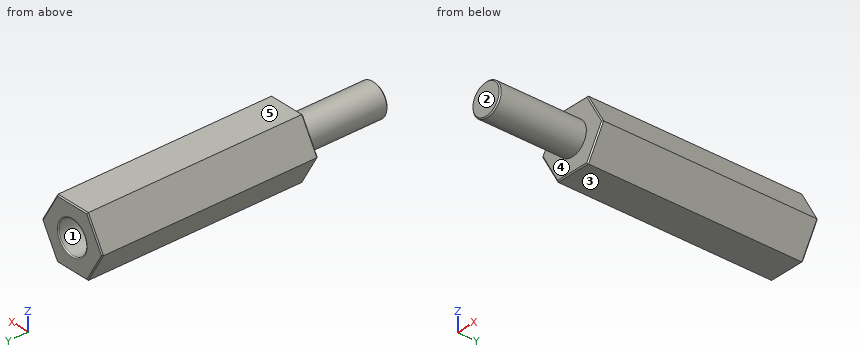
from build123d import *

# Parameters (mm, degrees)
BOSS_EXTRUDE1_DEPTH       = 20
SKETCH2_W                 = 1.5
SKETCH2_H                 = 8
F_3_0MM_DOWEL_HOLE1_D     = 3
F_3_0MM_DOWEL_HOLE1_DEPTH = 8
F_3_0MM_DOWEL_HOLE1_TIP   = 0.901290929
FILLET1_R                 = 0.1
CHAMFER1_SIZE             = 0.1


with BuildPart() as part:
    # Sketch1 → Boss-Extrude1 (new body)
    with BuildSketch(Plane.XZ):
        Polygon((-1.616580754, 2.8), (-3.233161507, 0), (-1.616580754, -2.8), (1.616580754, -2.8), (3.233161507, 0), (1.616580754, 2.8), align=None)
    extrude(amount=-BOSS_EXTRUDE1_DEPTH)

    # Sketch2 → Revolve1 (revolve)
    with BuildSketch(Plane.XY):
        with Locations((0.75, -4)):
            Rectangle(SKETCH2_W, SKETCH2_H)
    revolve(axis=Axis((0, 0, 0), (0, -1, 0)))

    # Ø3.0mm Dowel Hole1
    with Locations(Plane(origin=(0, 20, 0), x_dir=(1, 0, 0), z_dir=(0, 1, 0))):
        with Locations((0, 0)):
            Hole(F_3_0MM_DOWEL_HOLE1_D / 2, depth=F_3_0MM_DOWEL_HOLE1_DEPTH)
            with Locations((0, 0, -(F_3_0MM_DOWEL_HOLE1_DEPTH + F_3_0MM_DOWEL_HOLE1_TIP / 2))):  # 118° drill point
                Cone(0, F_3_0MM_DOWEL_HOLE1_D / 2, F_3_0MM_DOWEL_HOLE1_TIP, mode=Mode.SUBTRACT)

    # Fillet1
    fillet1_edges = [part.edges().sort_by_distance(p)[0] for p in [
        (1.5, 20, 0),
    ]]
    fillet(fillet1_edges, radius=FILLET1_R)

    # Chamfer1
    chamfer1_edges = [part.edges().sort_by_distance(p)[0] for p in [
        (-2.424871131, 20, -1.4),
        (0, 20, -2.8),
        (2.424871131, 20, -1.4),
        (2.424871131, 20, 1.4),
        (-1.5, -8, 0),
        (0, 20, 2.8),
        (2.424871131, 0, 1.4),
        (2.424871131, 0, -1.4),
        (0, 0, -2.8),
        (-2.424871131, 20, 1.4),
        (-2.424871131, 0, -1.4),
        (-2.424871131, 0, 1.4),
        (0, 0, 2.8),
    ]]
    chamfer(chamfer1_edges, length=CHAMFER1_SIZE)


solid = part.part
Geometry: final body of the model. Coordinates: model frame, mm. Face numbers are marked on the shaded views. A direction names the side the tool comes from. Give positions to 0.01 mm unless a question says otherwise; leave off trailing zeros. Loops run counter-clockwise (first coordinate to the right, second up) from the corner with the lowest first, then second, coordinate; pieces in that order, holes last. Notation, with made-up numbers: M 34,-11.75 L 61,-11.75 A20 ccw 61,22.25 Z; hole C 11,62 d10. An arc over 180 degrees is marked long. Put each result on its own line as item: value. Start each with the question number.
1) Cut plane C-C (z = -2.4). Output: boundary loops of the cut face in (x, y).
2) Contact query for flat-ended pins moving along their axis: pin 1 (1 mm diameter, centred on y = 11, z = -2, fed in from +X); pin 2 (2 mm diameter, centred on x = -2.5, z = -1.5, fed in from -Y); pin 3 (2 mm diameter, centred on y = 13, z = 0.5, fed in from -X). Output: stop coordinate, or through.
3) Access query for the marked faces 4 and 5. Directions: +Z, -Z, +X, -X, +Y, -Y. A direction counts if a zero-diameter tool reaches every point of the face in a straight line with its end or side. Return the directions, or none.
4) Pull-direction query (Z, two-part tool) for the marked faces 1, 2 and 3; classes: pulls with the +Z half, pulls with the -Z half, needs draft (parallel to the pull), parting line crosses it, or undercut.
5) Cut plane B-B (y = 1.5). Output: boundary loops of the cut face in (x, z).
6) Cut plane D-D (x = 2.75). Output: boundary loops of the cut face in (y, z), then the cut area to 3 significant figures.
7) Cut plane A-A (y = 15). Output: boundary loops of the cut face in (x, z), then the cut area to 3 significant figures.
8) Ray query, line 1 along Z through (x, y) = (0, 15.25); line 2 along X through (y, z) = (13, -0.95); line 3 along Y through (x, z) = (2.5, 0.95). Return the intervals inside material, ascending.
Verdict:
1. outline: M -1.85,0.1 L -1.73,0 L 1.73,0 L 1.85,0.1 L 1.85,19.9 L 1.73,20 L -1.73,20 L -1.85,19.9 Z
2. pin 1: x = 2.37
2. pin 2: y = 0
2. pin 3: x = -3.23
3. face 4: -Y
3. face 5: +Z, +X, -X, +Y, -Y
4. face 1: undercut
4. face 2: needs draft
4. face 3: pulls with the -Z half
5. outline: M -3.23,0 L -1.62,-2.8 L 1.62,-2.8 L 3.23,0 L 1.62,2.8 L -1.62,2.8 Z
6. outline: M 0,-0.64 L 0.1,-0.84 L 19.9,-0.84 L 20,-0.64 L 20,0.64 L 19.9,0.84 L 0.1,0.84 L 0,0.64 Z
6. area: 33.4 mm2
7. outline: M -3.23,0 L -1.62,-2.8 L 1.62,-2.8 L 3.23,0 L 1.62,2.8 L -1.62,2.8 Z; hole C 0,0 d3
7. area: 20.1 mm2
8. line 1: -2.8 to -1.5, 1.5 to 2.8
8. line 2: -2.68 to -1.16, 1.16 to 2.68
8. line 3: 0 to 20
